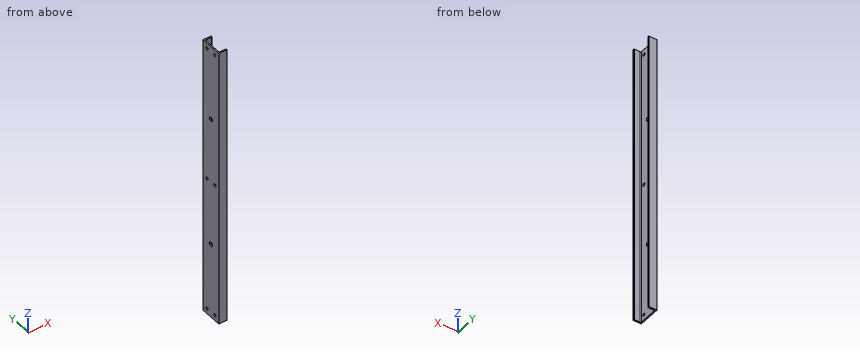
Autodesk Inventor part; units mm, degrees
ref_plane "YZ Plane" through (0, 0, 0) normal (1, 0, 0) x (0, 1, 0)
ref_plane "XZ Plane" through (0, 0, 0) normal (0, 1, 0) x (-1, 0, 0)
ref_plane "XY Plane" through (0, 0, 0) normal (0, 0, 1) x (1, 0, 0)
sketch "Sketch1" plane through (0, 0, 0) normal (0, 0, 1) x (1, 0, 0)
  line L0 (0, 25.4) -> (0, -25.4)
  line L1 (0, -25.4) -> (19.05, -25.4)
  line L2 (0, 25.4) -> (19.05, 25.4)
  line L3 (19.05, 25.4) -> (19.05, 22.225)
  line L4 (19.05, 22.225) -> (3.048, 22.225)
  line L5 (3.048, 22.225) -> (3.048, -22.225)
  line L6 (3.048, -22.225) -> (19.05, -22.225)
  line L7 (19.05, -22.225) -> (19.05, -25.4)
  point P0 (0, 0)
  point P1 (0, 0)
  dimension "d0" = 50.8
  dimension "d1" = 19.05
  dimension "d2" = 3.175
  dimension "d3" = 16.002
extrude "Extrusion1" add sketch "Sketch1" along normal mid plane 660.4
fillet "Fillet1" radius 1.5875 4 edges at (3.048, 22.225, 0) (3.048, -22.225, 0) (19.05, -22.225, 0) (19.05, 22.225, 0)
sketch "Sketch2" plane through (3.048, -20.6375, -330.2) normal (1, 0, 0) x (0, 0, -1)
  point P0 (-330.2, 20.6375)
  point P1 (-177.8, 20.6375)
  point P2 (-482.6, 20.6375)
  dimension "d7" = 304.8
  dimension "d8" = 152.4
hole "Hole1" at (3.048, 0, -152.4) at (3.048, 0, 152.4) direction (-1, 0, 0) diameter 9.525 depth 25.4 tip angle 118
sketch "Sketch3" plane through (3.048, -20.6375, -330.2) normal (1, 0, 0) x (0, 0, -1)
  circle A0 centre (-647.7, 33.3375) radius 12.7
  circle A1 centre (-647.7, 7.9375) radius 12.7
  circle A2 centre (-12.7, 33.3375) radius 12.7
  circle A3 centre (-12.7, 7.9375) radius 12.7
  circle A4 centre (-330.2, 33.3375) radius 12.7
  circle A5 centre (-330.2, 7.9375) radius 12.7
  point P0 (-330.2, 20.6375)
hole "Hole2" at (3.048, -12.7, -317.5) at (3.048, -12.7, 0) at (3.048, -12.7, 317.5) at (3.048, 12.7, 317.5) at (3.048, 12.7, 0) at (3.048, 12.7, -317.5) direction (-1, 0, 0) diameter 6.7564 depth 25.4 tip angle 118
equation "\"d4\" = Length"
equation "\"Length\" = 660.4"
properties part number "NASA-20-OP-01" material "Aluminum 6061"
For this review, take the finished solid that the model builds, in its own axes (mm). Round coordinates to 2 decimals unless told otherwise and drop trailing zeros. Write each loop counter-clockwise with the first axis right and the second up, starting at its lowest first coordinate (ties: lowest second). Pieces come first, ordered by that corner, then holes. Notation, with made-up numbers: (25.25, 71) - (53.25, 71) arc R21 ccw to (53.25, 94) - close; hole circle Ø6 at (72, 17). An arc over 180 degrees is marked (long way). Put each result on its own line as item: value.
Q1. We need section A-A (x = 9.5). Give the boundary of the cut face in (y, z) (3 decimals).
Solved:
outline: (-25.4, -330.2) - (-22.225, -330.2) - (-22.225, 330.2) - (-25.4, 330.2) - close; (22.225, -330.2) - (25.4, -330.2) - (25.4, 330.2) - (22.225, 330.2) - close
Q2. Wall thickness on probe 1 along Z at (x, y) = (1.25, 0); probe 2 along Z at (x, y) = (2.2, -12.7); probe 3 along Y at (x, z) = (2.2, 0): over which ranges is each line inside the solid? List them lowest first.
Solved:
probe 1: z = -330.2 to -157.16, -147.64 to 147.64, 157.16 to 330.2
probe 2: z = -330.2 to -320.88, -314.12 to -3.38, 3.38 to 314.12, 320.88 to 330.2
probe 3: y = -25.4 to -16.08, -9.32 to 9.32, 16.08 to 25.4
Q3. Insertion check: pin 1 Ø6 at (y, z) = (-12.7, 0) entering from +X; pin 2 Ø9 at (y, z) = (-12.7, 317.5) entering from +X. Each pin has a flat end and moves straight along its axis. Give the tip position at first contact, or say it passes through.
Solved:
pin 1: passes through
pin 2: stops at x = 3.05
